Work out the finished part from the listing and answer in its coordinate system (mm). Coordinates: 2 decimals unless noted, no trailing zeros. Write each loop counter-clockwise with the first axis right and the second up, starting at its lowest first coordinate (ties: lowest second). Pieces come first, ordered by that corner, then holes. Notation, with made-up numbers: (30.5, 5) - (63.5, 5) arc R20 ccw to (63.5, 18) - close; hole circle Ø8 at (21, 87). An arc over 180 degrees is marked (long way). Use CSV: the item, a comma, the result in double quotes. Start each with the question number.
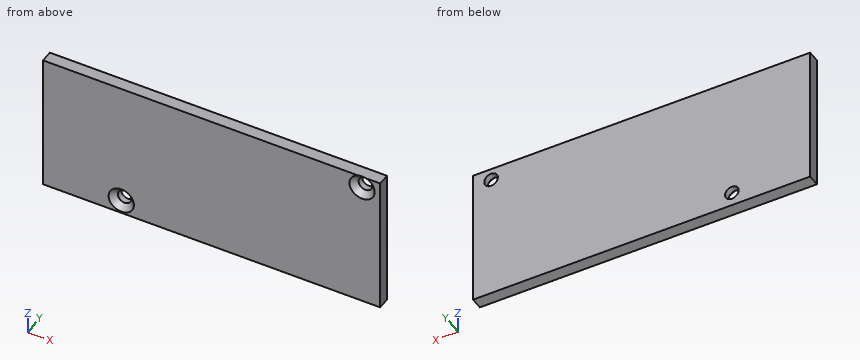
from build123d import *

# Parameters (mm, degrees)
SKETCH1_W                                      = 84
SKETCH1_H                                      = 35
BOSS_EXTRUDE1_DEPTH                            = 3
CSK_FOR_M3_FLAT_HEAD_MACHINE_SCREW1_AT_2_COUNT = 2
CSK_FOR_M3_FLAT_HEAD_MACHINE_SCREW1_AT_2_PITCH = 66.424769476


with BuildPart() as part:
    # Sketch1 → Boss-Extrude1 (new body)
    with BuildSketch(Plane(origin=(0, 0, 0), x_dir=(1, 0, 0), z_dir=(0, 1, 0))):
        Rectangle(SKETCH1_W, SKETCH1_H)
    extrude(amount=BOSS_EXTRUDE1_DEPTH)

    # Sketch5 → CSK for M3 Flat Head Machine Screw1 (revolve, cut)
    with BuildSketch(Plane(origin=(37.5, 0, 14.5), x_dir=(0, 0, -1), z_dir=(1, 0, 0))):
        Polygon((0, 0), (0, 3), (1.7, 3), (1.7, 1.45), (3.15, 0), align=None)
    csk_for_m3_flat_head_machine_screw1 = revolve(axis=Axis((37.5, -6.35, 14.5), (0, 1, 0)), mode=Mode.SUBTRACT)

    # CSK for M3 Flat Head Machine Screw1 at 2: CSK for M3 Flat Head Machine Screw1 ×2
    with Locations(*[Vector(-0.9032775043542898, 0, -0.4290568145682877) * (i * CSK_FOR_M3_FLAT_HEAD_MACHINE_SCREW1_AT_2_PITCH) for i in range(1, CSK_FOR_M3_FLAT_HEAD_MACHINE_SCREW1_AT_2_COUNT)]):
        add(csk_for_m3_flat_head_machine_screw1, mode=Mode.SUBTRACT)


solid = part.part
Item 1: A cutting plane is placed at B-B (x = 37.5). Determine the outline of the cut face in (y, z), then the cut area to 3 significant figures.
Item 2: A cutting plane is placed at C-C (x = -22.5). Determine the outline of the cut face in (y, z).
Item 3: A cutting plane is placed at A-A (z = 14.5). Determine the outline of the cut face in (x, y).
Item 4: Straight lines are drawn through the part: probe 1 along X at (y, z) = (2, -14); probe 2 along Z at (x, y) = (37.5, 2.7); probe 3 along X at (y, z) = (2.3, 14.5). For each, find the intervals that lie inside material, in ascending order. Write a range as [from, to].
Calculated:
1,outline,"(0, -17.5) - (3, -17.5) - (3, 12.8) - (1.45, 12.8) - (0, 11.35) - close; (0.15, 17.5) - (1.45, 16.2) - (3, 16.2) - (3, 17.5) - close"
1,area,"92.7 mm²"
2,outline,"(0, -17.5) - (3, -17.5) - (3, -15.7) - (1.45, -15.7) - (0, -17.15) - close; (0, -10.85) - (1.45, -12.3) - (3, -12.3) - (3, 17.5) - (0, 17.5) - close"
3,outline,"(-42, 0) - (34.35, 0) - (35.8, 1.45) - (35.8, 3) - (-42, 3) - close; (39.2, 1.45) - (40.65, 0) - (42, 0) - (42, 3) - (39.2, 3) - close"
4,probe 1,"x = [-42, -24.2], [-20.8, 42]"
4,probe 2,"z = [-17.5, 12.8], [16.2, 17.5]"
4,probe 3,"x = [-42, 35.8], [39.2, 42]"
